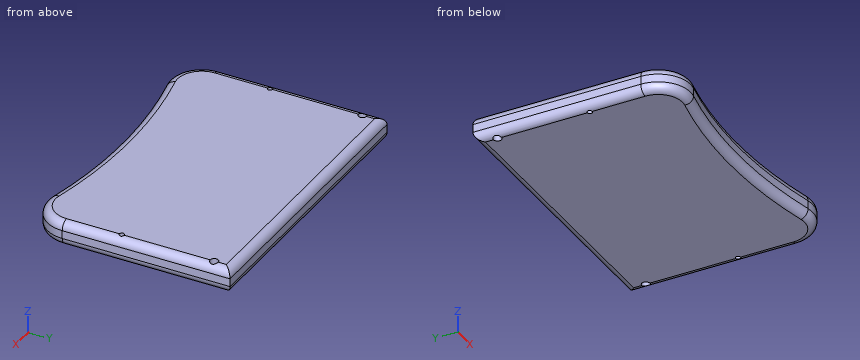
from build123d import *

# Parameters (mm, degrees)
F0_R         = 1.5
F0_R_2       = 2.5
F1_DEPTH     = 15
F2_T1_DEPTH  = 116.4597183962
F2_T3_DEPTH  = 205
F2_T6_ANGLE  = 102.5879293722
F2_T8_ANGLE  = 25.1758587444
F2_T10_ANGLE = 102.5879293722
F3_T1_DEPTH  = 205
F3_T3_DEPTH  = 116.4597183962
F3_T6_ANGLE  = 102.5879293722
F3_T8_ANGLE  = 25.1758587444
F3_T10_ANGLE = 102.5879293722


# Not quite as in the source:
# - a fillet or chamfer that OpenCascade refuses, or shapes differently, is made with other operations: its cross-section is extruded or revolved along the edge and cut away or added


with BuildPart() as f1:
    # F0 (on Top) → F1 (new body)
    with BuildSketch(Plane.XY):
        with BuildLine():
            Line((90, 69.696), (-90, 69.696))
            Line((-90, 69.696), (-90, -34.2637183962))
            ThreePointArc((-90, -34.2637183962), (-82.5064972072, -49.8710092439), (-65.6412472394, -53.7829723362))
            ThreePointArc((-65.6412472394, -53.7829723362), (0, -46.5431097607), (65.6412472394, -53.7829723362))
            ThreePointArc((65.6412472394, -53.7829723362), (82.5064972072, -49.8710092439), (90, -34.2637183962))
            Line((90, -34.2637183962), (90, 69.696))
        make_face()
        with Locations((-85, 0)):
            Circle(F0_R, mode=Mode.SUBTRACT)
        with Locations((85, 0)):
            Circle(F0_R, mode=Mode.SUBTRACT)
        with Locations((-85, 57.196)):
            Circle(F0_R_2, mode=Mode.SUBTRACT)
        with Locations((85, 57.196)):
            Circle(F0_R_2, mode=Mode.SUBTRACT)
    extrude(amount=F1_DEPTH)

    # F2: fillet of radius 5 on 2 edges, made by hand

    # F2_s2 → F2_t1 (cut)
    with BuildSketch(Plane.XZ.offset(-82.196)):
        with BuildLine():
            ThreePointArc((-90, 10), (-88.5355339059, 13.5355339059), (-85, 15))
            Line((-85, 15), (-90, 15))
            Line((-90, 15), (-90, 10))
        make_face()
        with BuildLine():
            ThreePointArc((90, 10), (88.5355339059, 13.5355339059), (85, 15))
            Line((85, 15), (90, 15))
            Line((90, 15), (90, 10))
        make_face()
    extrude(amount=F2_T1_DEPTH, mode=Mode.SUBTRACT)

    # F2_s4 → F2_t3 (cut)
    with BuildSketch(Plane.YZ.offset(-102.5)):
        with BuildLine():
            ThreePointArc((69.696, 10), (68.2315339059, 13.5355339059), (64.696, 15))
            Line((64.696, 15), (69.696, 15))
            Line((69.696, 15), (69.696, 10))
        make_face()
    extrude(amount=F2_T3_DEPTH, mode=Mode.SUBTRACT)

    # F2_s5 → F2_t6 (revolve, cut)
    with BuildSketch(Plane.XZ.offset(34.2637183962)):
        with BuildLine():
            ThreePointArc((-90, 10), (-88.5355339059, 13.5355339059), (-85, 15))
            Line((-85, 15), (-90, 15))
            Line((-90, 15), (-90, 10))
        make_face()
    revolve(axis=Axis((-70, -34.2637183962, 15), (0, 0, 1)), revolution_arc=F2_T6_ANGLE, mode=Mode.SUBTRACT)

    # F2_s7 → F2_t8 (revolve, cut)
    with BuildSketch(Plane(origin=(-73.9630818252, -16.5163478111, 0), x_dir=(0, 0, 1), z_dir=(-0.975962697, -0.217937638, 0))):
        with BuildLine():
            ThreePointArc((10, -38.1844763532), (13.5355339059, -36.7200102591), (15, -33.1844763532))
            Line((15, -33.1844763532), (15, -38.1844763532))
            Line((15, -38.1844763532), (10, -38.1844763532))
        make_face()
    revolve(axis=Axis((0, -347.7359089185, 15), (0, 0, -1)), revolution_arc=F2_T8_ANGLE, mode=Mode.SUBTRACT)

    # F2_s9 → F2_t10 (revolve, cut)
    with BuildSketch(Plane(origin=(73.9630818252, -16.5163478111, 0), x_dir=(0, 0, 1), z_dir=(-0.975962697, 0.217937638, 0))):
        with BuildLine():
            ThreePointArc((10, -38.1844763532), (13.5355339059, -36.7200102591), (15, -33.1844763532))
            Line((15, -33.1844763532), (15, -38.1844763532))
            Line((15, -38.1844763532), (10, -38.1844763532))
        make_face()
    revolve(axis=Axis((70, -34.2637183962, 15), (0, 0, 1)), revolution_arc=F2_T10_ANGLE, mode=Mode.SUBTRACT)

    # F3: fillet of radius 5 on 2 edges, made by hand

    # F3_s2 → F3_t1 (cut)
    with BuildSketch(Plane.YZ.offset(-102.5)):
        with BuildLine():
            ThreePointArc((64.696, 0), (68.2315339059, 1.4644660941), (69.696, 5))
            Line((69.696, 5), (69.696, 0))
            Line((69.696, 0), (64.696, 0))
        make_face()
    extrude(amount=F3_T1_DEPTH, mode=Mode.SUBTRACT)

    # F3_s4 → F3_t3 (cut)
    with BuildSketch(Plane.XZ.offset(-82.196)):
        with BuildLine():
            ThreePointArc((-85, 0), (-88.5355339059, 1.4644660941), (-90, 5))
            Line((-90, 5), (-90, 0))
            Line((-90, 0), (-85, 0))
        make_face()
        with BuildLine():
            ThreePointArc((85, 0), (88.5355339059, 1.4644660941), (90, 5))
            Line((90, 5), (90, 0))
            Line((90, 0), (85, 0))
        make_face()
    extrude(amount=F3_T3_DEPTH, mode=Mode.SUBTRACT)

    # F3_s5 → F3_t6 (revolve, cut)
    with BuildSketch(Plane.XZ.offset(34.2637183962)):
        with BuildLine():
            ThreePointArc((-85, 0), (-88.5355339059, 1.4644660941), (-90, 5))
            Line((-90, 5), (-90, 0))
            Line((-90, 0), (-85, 0))
        make_face()
    revolve(axis=Axis((-70, -34.2637183962, 0), (0, 0, 1)), revolution_arc=F3_T6_ANGLE, mode=Mode.SUBTRACT)

    # F3_s7 → F3_t8 (revolve, cut)
    with BuildSketch(Plane(origin=(-73.9630818252, -16.5163478111, 0), x_dir=(0, 0, 1), z_dir=(-0.975962697, -0.217937638, 0))):
        with BuildLine():
            ThreePointArc((0, -33.1844763532), (1.4644660941, -36.7200102591), (5, -38.1844763532))
            Line((5, -38.1844763532), (0, -38.1844763532))
            Line((0, -38.1844763532), (0, -33.1844763532))
        make_face()
    revolve(axis=Axis((0, -347.7359089185, 0), (0, 0, -1)), revolution_arc=F3_T8_ANGLE, mode=Mode.SUBTRACT)

    # F3_s9 → F3_t10 (revolve, cut)
    with BuildSketch(Plane(origin=(73.9630818252, -16.5163478111, 0), x_dir=(0, 0, 1), z_dir=(-0.975962697, 0.217937638, 0))):
        with BuildLine():
            ThreePointArc((5, -38.1844763532), (1.4644660941, -36.7200102591), (0, -33.1844763532))
            Line((0, -33.1844763532), (0, -38.1844763532))
            Line((0, -38.1844763532), (5, -38.1844763532))
        make_face()
    revolve(axis=Axis((70, -34.2637183962, 0), (0, 0, 1)), revolution_arc=F3_T10_ANGLE, mode=Mode.SUBTRACT)


solid = f1.part
Geometry: final body of the model. Coordinates: model frame, mm. Give positions to 0.01 mm unless a question says otherwise; leave off trailing zeros. Write each loop counter-clockwise with the first axis right and the second up, starting at its lowest first coordinate (ties: lowest second). Pieces come first, ordered by that corner, then holes. Notation, with made-up numbers: (-32, 80) -> (-21, 80) arc R37 cw to (-21, 117) -> close; hole circle Ø8 at (23, 8). An arc over 180 degrees is marked (long way). Answer as a JSON object with one key per item and string values.
1. Cut plane A-A on z = 3. Output: boundary loops of the cut face in (x, y), and give its area (3 significant figures).
Ans:
{"outline": "(-89.58, -34.26) arc R19.58 ccw to (-65.73, -53.38) arc R301.61 cw to (65.73, -53.38) arc R19.58 ccw to (89.58, -34.26) -> (89.58, 69.28) -> (-89.58, 69.28) -> close; hole circle Ø5 at (-85, 57.2); hole circle Ø3 at (-85, 0); hole circle Ø5 at (85, 57.2); hole circle Ø3 at (85, 0)", "area": "21,100 mm^2"}
2. Cut plane B-B on x = 0. Output: boundary loops of the cut face in (y, z), and give its area (3 significant figures).
Ans:
{"outline": "(-46.54, 5) arc R5 ccw to (-41.54, 0) -> (64.7, 0) arc R5 ccw to (69.7, 5) -> (69.7, 10) arc R5 ccw to (64.7, 15) -> (-41.54, 15) arc R5 ccw to (-46.54, 10) -> close", "area": "1,720 mm^2"}
3. Ray query, probe 1 along X at (y, z) = (57, 8.5); probe 2 along X at (y, z) = (58.5, 12.5); probe 3 along Y at (x, z) = (85, 12.25). Return the intervals inside material, ascending. Write a range as from..to.
Ans:
{"probe 1": "x = -90..-87.49, -82.51..82.51, 87.49..90", "probe 2": "x = -89.33..-87.13, -82.87..82.87, 87.13..89.33", "probe 3": "y = -46.67..-1.5, 1.5..54.7, 59.7..69.16"}
4. Contact query for flat-ended pins moving along their axis: pin 1 (2 mm diameter, centred on y = 16, z = 12, fed in from -X); pin 2 (2 mm diameter, centred on x = -9.5, z = 2, fed in from +Y); pin 3 (1 mm diameter, centred on x = 11.5, z = 13, fed in from +Y). Output: stop coordinate, or through.
Ans:
{"pin 1": "stops at x = -89.9", "pin 2": "stops at y = 69.28", "pin 3": "stops at y = 69.03"}
